from build123d import *

# Parameters (mm, degrees)
SKETCH18_R          = 1.905
SKETCH18_R_2        = 3.175
SKETCH18_R_3        = 6.35
SKETCH18_R_4        = 2.5
SKETCH18_R_5        = 10.922
BOSS_EXTRUDE4_DEPTH = 6.35
CHAMFER1_SIZE       = 2.54


with BuildPart() as part:
    # Sketch18 → Boss-Extrude4 (new body)
    with BuildSketch(Plane.XY):
        with BuildLine():
            Line((0, 0), (-265.604745697, 0))
            ThreePointArc((-265.604745697, 0), (-298.882523776, 76.131915965), (-307.699061234, 158.75))
            Line((-307.699061234, 158.75), (-307.699061234, 165.1))
            ThreePointArc((-307.699061234, 165.1), (-305.839189294, 169.590128061), (-301.349061234, 171.45))
            Line((-301.349061234, 171.45), (-231.499061234, 171.45))
            Line((-231.499061234, 171.45), (-159.473782125, 158.75))
            Line((-159.473782125, 158.75), (-28.014368889, 158.75))
            ThreePointArc((-28.014368889, 158.75), (-23.851207857, 157.194850386), (-21.727208485, 153.291130779))
            Line((-21.727208485, 153.291130779), (0, 0))
        make_face()
        with Locations((-180.594, 136.144)):
            Circle(SKETCH18_R, mode=Mode.SUBTRACT)
        with Locations((-11.423473622, 24.034728138)):
            Circle(SKETCH18_R_2, mode=Mode.SUBTRACT)
        with Locations((-27.253356194, 124.406511892)):
            Circle(SKETCH18_R_2, mode=Mode.SUBTRACT)
        with Locations((-35.200938766, 146.05)):
            Circle(SKETCH18_R_3, mode=Mode.SUBTRACT)
        with Locations((-301.900938766, 146.05)):
            Circle(SKETCH18_R_2, mode=Mode.SUBTRACT)
        with Locations((-301.569673588, 132.761391752)):
            Circle(SKETCH18_R_2, mode=Mode.SUBTRACT)
        with Locations((-300.579872803, 119.537524267)):
            Circle(SKETCH18_R_2, mode=Mode.SUBTRACT)
        with Locations((-298.943543444, 106.442822899)):
            Circle(SKETCH18_R_2, mode=Mode.SUBTRACT)
        with Locations((-239.568937637, 24.034728138)):
            Circle(SKETCH18_R_2, mode=Mode.SUBTRACT)
        with Locations((-286.962142025, 164.850708953)):
            Circle(SKETCH18_R_2, mode=Mode.SUBTRACT)
        with Locations((-187.097045256, 107.95)):
            Circle(SKETCH18_R_4, mode=Mode.SUBTRACT)
        with Locations((-180.594, 105.156)):
            Circle(SKETCH18_R, mode=Mode.SUBTRACT)
        with Locations((-165.1, 120.65)):
            Circle(SKETCH18_R_5, mode=Mode.SUBTRACT)
        with Locations((-165.1, 146.05)):
            Circle(SKETCH18_R_4, mode=Mode.SUBTRACT)
        with Locations((-149.606, 105.156)):
            Circle(SKETCH18_R, mode=Mode.SUBTRACT)
        with Locations((-149.606, 136.144)):
            Circle(SKETCH18_R, mode=Mode.SUBTRACT)
        with Locations((-143.102954744, 107.95)):
            Circle(SKETCH18_R_4, mode=Mode.SUBTRACT)
    extrude(amount=BOSS_EXTRUDE4_DEPTH)

    # Chamfer1
    chamfer1_edges = [part.edges().sort_by_distance(p)[0] for p in [
        (-14.598473622, 24.034728138, 0),
        (-30.428356194, 124.406511892, 0),
        (-242.743937637, 24.034728138, 0),
        (-290.137142025, 164.850708953, 0),
    ]]
    chamfer(chamfer1_edges, length=CHAMFER1_SIZE)


solid = part.part
Could you check a few things on this model? Use its own coordinates, in mm. A direction names the side the tool comes from. Give positions to 0.01 mm unless a question says otherwise; leave off trailing zeros. Order: outer loops, then holes, each group sorted by start corner. A loop starts at its lowest first (then second) coordinate and runs counter-clockwise, first axis right, second up. Notation, with made-up numbers: (62, -33) - (102, -33) arc R20 ccw to (102, -10) - close; hole circle Ø9 at (7.5, -23). An arc over 180 degrees is marked (long way). One line per question, with ' | ' between items. Start each with the question number.
Item 1: Thinking about a two-plate mould opening in Y: for faces 4 (the flat face through (-195.99, 165.19, 3.13)), 5 (the flat face through (-131, 0, 3)), 6 (the cylindrical face through (-24.32, 123.19, 4.42)), which applies, pulls with the +Y half, pulls with the -Y half, needs draft (parallel to the pull), parting line crosses it, or undercut?
Item 2: I want a section at B-B on z = 3.75. Give the number of separate pieces and of enclosed holes in the cut face, then the cut area to 3 significant figures.
Item 3: I want a section at C-C on y = 52. Write out the boundary of the cut face in (x, z), then the cut area to 3 significant figures.
Item 4: I want a section at A-A on x = -113. Write out the boundary of the cut face in (y, z), then the cut area to 3 significant figures.
Item 5: I need wall thicknesses on probe 1 along X at (y, z) = (20, 0.75); probe 2 along X at (y, z) = (124, 2.5); probe 3 along Y at (x, z) = (-147, 3). Which ranges of each line are inside material? Lowest first, please. Write a range as [from, to].
Item 6: I'm going to push flat-ended pins straight in: pin 1 Ø3 at (y, z) = (161, 2.5) entering from -X; pin 2 Ø3 at (x, y) = (-149.606, 105.156) entering from +Z; pin 3 Ø1.5 at (y, z) = (67.5, 3.5) entering from -X; pin 4 Ø1 at (y, z) = (116, 3) entering from +X. Where does each tip first touch, or does it pass through?
Item 7: For faces 1 (the flat face through (-307.699, 162, 3)), 2 (the flat face through (-95, 158.75, 3)), 3 (the cylindrical face through (-303.75, 119.68, 3.13)), which set-ups out of +Z, -Z, +X, -X, +Y, -Y let a thin tool reach every point of the face, with its end or its side?
Verdict:
1) face 4: pulls with the +Y half | face 5: pulls with the -Y half | face 6: undercut
2) separate pieces: 1 | enclosed holes: 17 | area: 45,700 mm^2
3) outline: (-291.27, 0) - (-7.37, 0) - (-7.37, 6.35) - (-291.27, 6.35) - close | area: 1,800 mm^2
4) outline: (0, 0) - (158.75, 0) - (158.75, 6.35) - (0, 6.35) - close | area: 1,010 mm^2
5) probe 1: [-277.13, -242.46], [-236.68, -14.32], [-8.53, -2.83] | probe 2: [-307.1, -175.5], [-154.7, -30.44], [-24.06, -17.58] | probe 3: [0, 158.75]
6) pin 1: x = -307.7 | pin 2: through | pin 3: x = -296.67 | pin 4: x = -16.37
7) face 1: +Z, -Z, -X, +Y | face 2: +Z, -Z, +X, +Y | face 3: +Z, -Z
